Autodesk Inventor part; units mm, degrees
ref_plane "YZ Plane" through (0, 0, 0) normal (1, 0, 0) x (0, 1, 0)
ref_plane "XZ Plane" through (0, 0, 0) normal (0, 1, 0) x (-1, 0, 0)
ref_plane "XY Plane" through (0, 0, 0) normal (0, 0, 1) x (1, 0, 0)
sketch "Sketch1" plane through (0, 0, 0) normal (0, 0, 1) x (1, 0, 0)
  line L0 (-0.0471, -0.0824) -> (104.8002, -0.0824) construction
  line L1 (104.8002, -0.0824) -> (104.8002, -53.0533) construction
  line L2 (104.8002, -53.0533) -> (-0.0471, -53.0533) construction
  line L3 (-0.0471, -53.0533) -> (-0.0471, -0.0824) construction
  line L4 (48.7, -18.9324) -> (48.7, -0.9324)
  line L5 (56.7, -0.9324) -> (57.6, -17.9324)
  line L6 (57.6, -36.0324) -> (57.6, -50.0324)
  line L7 (48.7, -50.0324) -> (57.6, -50.0324)
  line L8 (56.7, -0.9324) -> (48.7, -0.9324)
  line L9 (48.7, -18.9324) -> (52.7, -22.9324)
  line L10 (52.7, -22.9324) -> (52.7, -28.5324)
  line L11 (52.7, -28.5324) -> (48.7, -32.5324)
  line L12 (57.6, -36.0324) -> (63.4, -30.2324)
  line L13 (63.4, -30.2324) -> (63.4, -23.1492)
  line L14 (63.4, -23.1492) -> (57.6, -17.9324)
  line L15 (48.7, -32.5324) -> (48.7, -50.0324)
  point P0 (0, 0)
  dimension "d19" = 49.1
  dimension "d44" = 8
  dimension "d68" = 48.7
  dimension "d74" = 135
  dimension "d77" = 135
  dimension "d82" = 0.9
  dimension "d85" = 10.7
  dimension "d86" = 135
  dimension "d87" = 135
  dimension "d96" = 0.85
  dimension "d104" = 18
  dimension "d105" = 17.5
  dimension "d117" = 8.9
  dimension "d120" = 14
  dimension "d121" = 17
  dimension "d124" = 4
extrude "Extrusion2" add sketch "Sketch1" along normal blind 18
fillet "Fillet3" radius 2 4 edges at (56.7, -0.9324, 9) (48.7, -0.9324, 9) (57.6, -50.0324, 9) (48.7, -50.0324, 9)
fillet "Fillet4" radius 4 8 edges at (48.7, -18.9324, 9) (57.6, -17.9324, 9) (52.7, -22.9324, 9) (52.7, -28.5324, 9) (48.7, -32.5324, 9) (57.6, -36.0324, 9) (63.4, -30.2324, 9) (63.4, -23.1492, 9)
sketch "Sketch2" plane through (48.7, -48.0324, 0) normal (-1, 0, 0) x (0, 0, 1)
  line L0 (0, 0) -> (0, 13.8431)
  line L1 (18, 13.8431) -> (18, 0)
  line L2 (0, -2) -> (18, -2)
  line L3 (5, 1.1) -> (5, 7.9) construction
  line L4 (7.25, 1.1) -> (7.25, 7.9)
  line L5 (2.75, 7.9) -> (2.75, 1.1)
  arc A0 (2.75, 1.1) -> (7.25, 1.1) centre (5, 1.1) ccw
  arc A1 (7.25, 7.9) -> (2.75, 7.9) centre (5, 7.9) ccw
  line L6 (13, 7.9) -> (13, 1.1) construction
  line L7 (10.75, 7.9) -> (10.75, 1.1)
  line L8 (15.25, 1.1) -> (15.25, 7.9)
  arc A2 (15.25, 7.9) -> (10.75, 7.9) centre (13, 7.9) ccw
  arc A3 (10.75, 1.1) -> (15.25, 1.1) centre (13, 1.1) ccw
  point P0 (0, 48.0324)
  point P1 (5, 4.5)
  point P2 (13, 4.5)
  dimension "d129" = 4.5
  dimension "d130" = 6.8
  dimension "d131" = 3.1
  dimension "d132" = 5
  dimension "d133" = 5
sketch "Sketch3" plane through (57.6, -48.0324, 18) normal (1, 0, 0) x (0, 0, -1)
  line L0 (5, 7.9) -> (5, 1.1) construction
  line L1 (13, 1.1) -> (13, 7.9) construction
  line L2 (5, 4.1) -> (5, 6.6) construction
  line L3 (7.25, 4.1) -> (7.25, 6.6)
  line L4 (2.75, 6.6) -> (2.75, 4.1)
  arc A0 (2.75, 4.1) -> (7.25, 4.1) centre (5, 4.1) ccw
  arc A1 (7.25, 6.6) -> (2.75, 6.6) centre (5, 6.6) ccw
  line L5 (13, 4.1) -> (13, 6.6) construction
  line L6 (10.75, 4.1) -> (10.75, 6.6)
  line L7 (15.25, 6.6) -> (15.25, 4.1)
  arc A2 (10.75, 4.1) -> (15.25, 4.1) centre (13, 4.1) ccw
  arc A3 (15.25, 6.6) -> (10.75, 6.6) centre (13, 6.6) ccw
  line L8 (0, -2) -> (18, -2)
  point P0 (18, 48.0324)
  point P1 (5, 5.35)
  point P2 (13, 5.35)
  dimension "d134" = 2.5
  dimension "d135" = 4.5
  dimension "d136" = 6.1
loft "Loft1" cut profiles "Sketch2", "Sketch3" contours A0 L5 A1 L4 / L6 A3 L7 A2
loft "Loft2" cut profiles "Sketch2", "Sketch3" contours A2 L8 A3 L7 / A0 L4 A1 L3
sketch "Sketch4" plane through (0, 0, 0) normal (0, 0, -1) x (-1, 0, 0)
  line L0 (-63.4, -24.9314) -> (-63.4, -28.5756)
  line L1 (-50.7, -0.9324) -> (-54.8031, -0.9324)
  point P0 (0, 0)
  point P1 (-58.4, -26.6324)
  dimension "d145" = 25.7
  dimension "d146" = 5
hole "Hole1" at (58.4, -26.6324, 0) direction (0, 0, 1) diameter 4.5 end through all
properties part number "ExtruderSatoerCamArm"
Model file for the job. Use its own axes, mm. A direction names the side the tool comes from. Give positions to 0.01 mm unless a question says otherwise; leave off trailing zeros. Order: outer loops, then holes, each group sorted by start corner. A loop starts at its lowest first (then second) coordinate and runs counter-clockwise, first axis right, second up. Notation, with made-up numbers: M 55.5,29.5 L 72.5,29.5 A26 ccw 72.5,45.5 Z; hole C 61.25,-6.5 d9. An arc over 180 degrees is marked long. Put each result on its own line as item: value. Start each with the question number.
(1) Drill centre lines: L1, parallel to Y at x = 60, z = 14.75; L2, parallel to X at y = -28.5, z = 6; L3, parallel to Y at x = 58.4, z = 3.5. Where is each one in solid material? Low to high. Write a range as [from, to].
(2) Pull direction Y, two halves, no side cores. Call faces 3 (the face through (52.4, -28.4, 9.1)), 4 (the face through (57.913, -36.138, 9.126)), 5 (the face through (54, -25, 18)): released by +Y, released by -Y, zero draft, split by the parting line, or undercut.
(3) Band-saw the part on A-A on z = 2. Give the cut face in (x, y).
(4) Pin check, flat tips, straight feed: pin 1 Ø5 at (x, y) = (58.4, -26.63) entering from -Z; pin 2 Ø1.5 at (x, z) = (58, 14.5) entering from -Y; pin 3 Ø6 at (y, z) = (-37, 13) entering from +X; pin 4 Ø8.5 at (y, z) = (-45.5, 10.5) entering from +X. Stop position of each tip, or through.
(5) Tool access for faces 1 (the face through (52.404, -23.079, 9.126)), 2 (the face through (56.2, -1.5, 9.1)): list every direction of +Z, -Z, +X, -X, +Y, -Y with a clear straight run to the whole face (end or side of a thin tool).
(6) Band-saw the part on C-C on z = 13.5. Count the separate pieces of the cut face and the enclosed holes in it, then the cut area to 3 significant figures.
(7) Band-saw the part on B-B on y = -25.5. Give the cut face in (x, z), then the cut area to 3 significant figures.
Results below:
1. L1: y = [-33.63, -28.21], [-25.05, -20.09]
1. L2: x = [52.36, 57.15], [59.65, 63.4]
1. L3: y = [-35.29, -28.88], [-24.38, -18.59]
2. face 3: undercut
2. face 4: released by -Y
2. face 5: zero draft
3. outline: M 48.7,-48.03 A2 ccw 50.7,-50.03 L 55.6,-50.03 A2 ccw 57.6,-48.03 L 57.6,-37.69 A4 cw 58.77,-34.86 L 62.23,-31.4 A4 ccw 63.4,-28.58 L 63.4,-24.93 A4 ccw 62.07,-21.96 L 58.83,-19.04 A4 cw 57.51,-16.28 L 56.8,-2.83 A2 ccw 54.8,-0.93 L 50.7,-0.93 A2 ccw 48.7,-2.93 L 48.7,-17.28 A4 ccw 49.87,-20.1 L 51.53,-21.76 A4 cw 52.7,-24.59 L 52.7,-26.88 A4 cw 51.53,-29.7 L 49.87,-31.36 A4 ccw 48.7,-34.19 Z; hole C 58.4,-26.63 d4.5
4. pin 1: stops at z = 0
4. pin 2: stops at y = -49.16
4. pin 3: stops at x = 59.63
4. pin 4: stops at x = 57.6
5. face 1: +Z, -Z, -X
5. face 2: +Z, -Z, +X, +Y
6. separate pieces: 2
6. enclosed holes: 1
6. area: 364 mm2
7. outline: M 52.7,0 L 56.46,0 L 56.46,18 L 52.7,18 Z; M 60.34,0 L 63.4,0 L 63.4,18 L 60.34,18 Z
7. area: 123 mm2
